```python
from build123d import *

# Parameters (mm, degrees)
SKETCH_1_W          = 100
SKETCH_1_H          = 19.6
EXTRUDE_1_DEPTH     = 19.6
SKETCH_3_W          = 41
SKETCH_3_H          = 19.6
CUT_EXTRUDE_1_DEPTH = 10
SKETCH_6_W          = 20
SKETCH_6_H          = 19.6
CUT_EXTRUDE_2_DEPTH = 15.5
SKETCH_22_W         = 20
SKETCH_22_H         = 9.8
EXTRUDE_4_DEPTH     = 10
SHELL_3_T           = -2
SKETCH_23_W         = 15.6
SKETCH_23_H         = 15.6
EXTRUDE_5_DEPTH     = 0.5


with BuildPart() as part:
    # 草圖1 → 填料-伸長1 (new body)
    with BuildSketch(Plane.XY):
        Rectangle(SKETCH_1_W, SKETCH_1_H)
    extrude(amount=EXTRUDE_1_DEPTH)

    # 草圖3 → 除料-伸長1 (cut)
    with BuildSketch(Plane(origin=(0, 9.8, 0), x_dir=(1, 0, 0), z_dir=(0, 1, 0))):
        with Locations((0, -9.8)):
            Rectangle(SKETCH_3_W, SKETCH_3_H)
    extrude(amount=-CUT_EXTRUDE_1_DEPTH, mode=Mode.SUBTRACT)

    # 草圖6 → 除料-伸長2 (cut)
    with BuildSketch(Plane(origin=(0, -0.2, 0), x_dir=(1, 0, 0), z_dir=(0, 1, 0))):
        Rectangle(SKETCH_6_W, SKETCH_6_H)
    extrude(amount=-CUT_EXTRUDE_2_DEPTH, mode=Mode.SUBTRACT)

    # 草圖22 → 填料-伸長4 (add)
    with BuildSketch(Plane(origin=(0, -0.2, 0), x_dir=(1, 0, 0), z_dir=(0, 1, 0))):
        with Locations((0, -14.7)):
            Rectangle(SKETCH_22_W, SKETCH_22_H)
    extrude(amount=EXTRUDE_4_DEPTH)

    # 薄殼3
    shell_3_openings = [part.faces().sort_by_distance(p)[0] for p in [
        (-50, 0, 9.8),
    ]]
    offset(amount=SHELL_3_T, openings=shell_3_openings, kind=Kind.INTERSECTION)

    # 草圖23 → 填料-伸長5 (add)
    with BuildSketch(Plane.ZY.offset(50)):
        with Locations((9.8, 0)):
            Rectangle(SKETCH_23_W, SKETCH_23_H)
    extrude(amount=-EXTRUDE_5_DEPTH)


solid = part.part
```
Can you work these out from the model? Positions are in its coordinate system, mm. A direction names the side the tool comes from. Coordinates: 2 decimals unless noted, no trailing zeros. Write each loop counter-clockwise with the first axis right and the second up, starting at its lowest first coordinate (ties: lowest second). Pieces come first, ordered by that corner, then holes. Notation, with made-up numbers: (22, -23) - (61, -23) arc R10 cw to (61, -18) - close; hole circle Ø1 at (73, 27.5). An arc over 180 degrees is marked (long way). Return JSON: item names as keys, results as strings.
Q1. If we section it at C-C (x = -28): Please give me the cut outline in (y, z).
Computed values:
{"outline": "(-9.8, 0) - (9.8, 0) - (9.8, 19.6) - (-9.8, 19.6) - close; hole (-7.8, 2) - (7.8, 2) - (7.8, 17.6) - (-7.8, 17.6) - close"}
Q2. On a 3-axis mill with a long thin cutter (end or side, diameter ignored), from which of +Z, -Z, +X, -X, +Y, -Y can I reach the whole of each face in a straight line? I mean faces 1 (the flat face through (-50, 0, 10)), 2 (the flat face through (48, 0, 10)), 3 (the flat face through (-10, 5, 15)). Say none if no direction works.
Computed values:
{"face 1": "+Z, -Z, -X, +Y, -Y", "face 2": "none", "face 3": "+Z, -Z, +Y"}
Q3. If we section it at B-B (z = 4.5): Please give me the cut outline in (x, y), then the cut area to 3 significant figures.
Computed values:
{"outline": "(-50, -9.8) - (-10, -9.8) - (-10, -0.2) - (-20.5, -0.2) - (-20.5, 9.8) - (-50, 9.8) - close; (10, -9.8) - (50, -9.8) - (50, 9.8) - (20.5, 9.8) - (20.5, -0.2) - (10, -0.2) - close; hole (-49.5, -7.8) - (-12, -7.8) - (-12, -2.2) - (-22.5, -2.2) - (-22.5, 7.8) - (-49.5, 7.8) - close; hole (12, -7.8) - (48, -7.8) - (48, 7.8) - (22.5, 7.8) - (22.5, -2.2) - (12, -2.2) - close", "area": "421 mm2"}
Q4. Thinking about a two-plate mould opening in Z: for faces 4 (the flat face through (0, 0, 9.8)), 5 (the flat face through (0, 7.8, 15)), 6 (the flat face through (-15, -0.2, 10)), 7 (the flat face through (17, -2.2, 10)), which applies, +Z half, -Z half, draft (parallel to the pull), parting line (faces both ways), or undercut?
Computed values:
{"face 4": "-Z half", "face 5": "undercut", "face 6": "draft", "face 7": "undercut"}
Q5. Please list where these lines run through material, in increasing order: L1, parallel to X at y = 7, z = 14.75; L2, parallel to X at y = 8.5, z = 12.75; L3, parallel to X at y = -1, z = 7.5. Write a range as from..to.
Computed values:
{"L1": "x = -50..-49.5, -22.5..-20.5, -10..-8, 8..10, 20.5..22.5, 48..50", "L2": "x = -50..-20.5, -10..10, 20.5..50", "L3": "x = -50..-49.5, -22.5..-10, 10..22.5, 48..50"}
Q6. If we section it at A-A (y = 2.75): Please give me the cut outline in (x, z), then the cut area to 3 significant figures.
Computed values:
{"outline": "(-50, 0) - (-20.5, 0) - (-20.5, 19.6) - (-50, 19.6) - close; (-10, 9.8) - (10, 9.8) - (10, 19.6) - (-10, 19.6) - close; (20.5, 0) - (50, 0) - (50, 19.6) - (20.5, 19.6) - close; hole (-49.5, 2) - (-22.5, 2) - (-22.5, 17.6) - (-49.5, 17.6) - close; hole (-8, 11.8) - (8, 11.8) - (8, 17.6) - (-8, 17.6) - close; hole (22.5, 2) - (48, 2) - (48, 17.6) - (22.5, 17.6) - close", "area": "441 mm2"}
Q7. I'm going to push flat-ended pins straight in: pin 1 Ø1 at (x, y) = (-14.5, 2) entering from -Z; pin 2 Ø6 at (x, y) = (-5, 1) entering from -Z. Where does each tip first touch, or does it pass through?
Computed values:
{"pin 1": "passes through", "pin 2": "stops at z = 9.8"}
Q8. If we section it at D-D (y = -5.75): Please give me the cut outline in (x, z), then the cut area to 3 significant figures.
Computed values:
{"outline": "(-50, 0) - (-10, 0) - (-10, 9.8) - (10, 9.8) - (10, 0) - (50, 0) - (50, 19.6) - (-50, 19.6) - close; hole (-49.5, 2) - (-12, 2) - (-12, 11.8) - (12, 11.8) - (12, 2) - (48, 2) - (48, 17.6) - (-49.5, 17.6) - close", "area": "478 mm2"}
